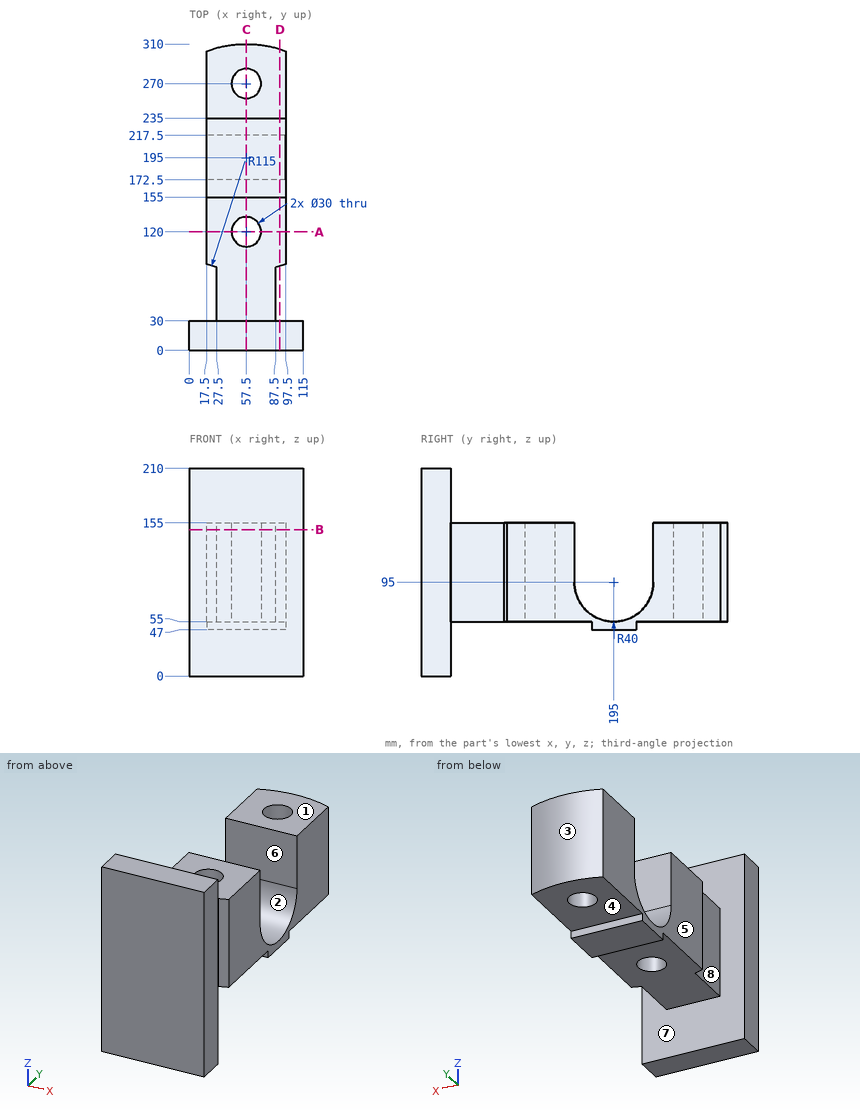
Answer from the drawing. Dimensions are ordinates in mm from the lowest x, y and z of the part. A direction names the side the tool comes from. Round coordinates to 2 decimals unless told otherwise and drop trailing zeros. Write each loop counter-clockwise with the first axis right and the second up, starting at its lowest first coordinate (ties: lowest second). Pieces come first, ordered by that corner, then holes.
1. Which of the six approach directions +Z, -Z, +X, -X, +Y, -Y give full straight-line access (tool end or side, diameter ignored) to the marked faces 4, 5, 6, 7 and 8?
2. The part is cut by section B-B, the plane z = 148. Determine the outline of the cut face in (x, y).
3. Determine the mould class of the marked faces 1, 2 and 3 for opening direction Y: pulls with the +Y half, pulls with the -Y half, needs draft (parallel to the pull), parting line crosses it, or undercut.
4. The part is cut by section A-A, the plane y = 120. Determine the outline of the cut face in (x, z).
5. The part is cut by section C-C, the plane x = 57.5. Determine the outline of the cut face in (y, z), then the cut area to 3 significant figures.
6. Straight lines are drawn through the part: L1, parallel to Y at x = 57.5, z = 133; L2, parallel to Y at x = 38.5, z = 46; L3, parallel to Z at x = 44.5, y = 32. For each, find the intervals that lie inside material, in ascending order.
7. Given pin 1 Ø9 at (x, z) = (70.5, 49.5) entering from +Y; pin 2 Ø18 at (x, z) = (75.5, 129) entering from +Y; pin 3 Ø6 at (y, z) = (67, 77.5) entering from -X; pin 4 Ø18 at (x, y) = (57.5, 120) entering from +Z, each flat-ended and moving along its own axis, determine where each tip first touches the part or whether it passes through.
8. The part is cut by section D-D, the plane x = 91.5. Determine the outline of the cut face in (y, z), then the cut area to 3 significant figures.
Values:
1. face 4: -Z, +X, -X, +Y
1. face 5: +Z, -Z, -X, +Y
1. face 6: +Z, +X, -X
1. face 7: none
1. face 8: +Z, -Z, -X
2. outline: (0, 0) - (115, 0) - (115, 30) - (87.5, 30) - (87.5, 83.98) arc R115 ccw to (97.5, 87.18) - (97.5, 155) - (17.5, 155) - (17.5, 87.18) arc R115 ccw to (27.5, 83.98) - (27.5, 30) - (0, 30) - close; (17.5, 235) - (97.5, 235) - (97.5, 302.82) arc R115 ccw to (17.5, 302.82) - close; hole circle Ø30 at (57.5, 120); hole circle Ø30 at (57.5, 270)
3. face 1: needs draft
3. face 2: undercut
3. face 3: pulls with the +Y half
4. outline: (17.5, 55) - (42.5, 55) - (42.5, 155) - (17.5, 155) - close; (72.5, 55) - (97.5, 55) - (97.5, 155) - (72.5, 155) - close
5. outline: (0, 0) - (30, 0) - (30, 55) - (105, 55) - (105, 155) - (30, 155) - (30, 210) - (0, 210) - close; (135, 55) - (172.5, 55) - (172.5, 47) - (217.5, 47) - (217.5, 55) - (255, 55) - (255, 155) - (235, 155) - (235, 95) arc R40 cw to (155, 95) - (155, 155) - (135, 155) - close; (285, 55) - (310, 55) - (310, 155) - (285, 155) - close
5. area: 21,300 mm2
6. L1: y = 0 to 105, 135 to 155, 235 to 255, 285 to 310
6. L2: y = 0 to 30
6. L3: z = 55 to 155
7. pin 1: stops at y = 217.5
7. pin 2: stops at y = 309.65
7. pin 3: stops at x = 27.5
7. pin 4: passes through
8. outline: (0, 0) - (30, 0) - (30, 210) - (0, 210) - close; (85.14, 55) - (172.5, 55) - (172.5, 47) - (217.5, 47) - (217.5, 55) - (304.86, 55) - (304.86, 155) - (235, 155) - (235, 95) arc R40 cw to (155, 95) - (155, 155) - (85.14, 155) - close
8. area: 21,300 mm2
